from build123d import *

# Parameters (mm, degrees)
F1_DEPTH = 76.1175008
F2_R     = 1.98374
F3_R     = 3.69316
F4_R     = 1.8288
F5_DEPTH = 1.70942
F6_R     = 0.762
F7_W     = 6
F7_H     = 3.175
F8_DEPTH = 1.70942


# Not quite as in the source:
# - a feature names something its author has since deleted; it is built from what else it names


with BuildPart() as f1:
    # F0 (on Top) → F1 (new body)
    with BuildSketch(Plane.XY):
        Polygon((-1.70942, 0), (0, 0), (0, 16.7533828), (28.6143954, 16.7533828), (28.6143954, 31.2090308), (26.9049754, 31.2090308), (26.9049754, 18.4628028), (-1.70942, 18.4628028), align=None)
    extrude(amount=F1_DEPTH)

    # F2
    f2_edges = [f1.edges().sort_by_distance(p)[0] for p in [
        (0, 16.753383, 38.05875),
        (26.904975, 18.462803, 38.05875),
    ]]
    fillet(f2_edges, radius=F2_R)

    # F3
    f3_edges = [f1.edges().sort_by_distance(p)[0] for p in [
        (-1.70942, 18.462803, 38.05875),
        (28.614395, 16.753383, 38.05875),
    ]]
    fillet(f3_edges, radius=F3_R)

    # F4 (on face) → F5 (cut, through all)
    with BuildSketch(Plane.XZ.offset(-16.7533828)):
        with Locations((20.9524854, 72.1487508)):
            Circle(F4_R)
        with Locations((20.9524854, 38.0587504)):
            Circle(F4_R)
        with Locations((20.9524854, 3.96875)):
            Circle(F4_R)
    extrude(amount=-F5_DEPTH, mode=Mode.SUBTRACT)

    # F6
    f6_edges = [f1.edges().sort_by_distance(p)[0] for p in [
        (-0.85471, 0, 76.117501),
        (-0.85471, 0, 0),
    ]]
    fillet(f6_edges, radius=F6_R)

    # F7 (on face) → F8 (cut, through all)
    with BuildSketch(Plane(origin=(26.9049754, 0, 0), x_dir=(0, -1, 0), z_dir=(-1, 0, 0))):
        with Locations((-25.0340308, 71.3550008)):
            Rectangle(F7_W, F7_H)
        with Locations((-25.0340308, 4.7625)):
            Rectangle(F7_W, F7_H)
    extrude(amount=-F8_DEPTH, mode=Mode.SUBTRACT)


solid = f1.part
For this review, take the finished solid that the model builds, in its own axes (mm). A direction names the side the tool comes from. Give positions to 0.01 mm unless a question says otherwise; leave off trailing zeros. Order: outer loops, then holes, each group sorted by start corner. A loop starts at its lowest first (then second) coordinate and runs counter-clockwise, first axis right, second up. Notation, with made-up numbers: (-6, -19) - (40, -19) arc R16 ccw to (40, 5) - close; hole circle Ø10 at (-30.5, 42). An arc over 180 degrees is marked (long way). Answer as a JSON object with one key per item and string values. Group by question number.
Item 1: Take a section at D-D on x = 10.5. Give the boundary of the cut face in (y, z).
Item 2: Clearance check with flat-ended pins moving along their axes: pin 1 Ø1.9 at (x, z) = (28, 72) entering from -Y; pin 2 Ø5 at (x, y) = (15.5, 21.5) entering from +Z; pin 3 Ø11.5 at (x, z) = (16.5, 46) entering from +Y; pin 4 Ø5.5 at (y, z) = (26, 21.5) entering from -X (3 decimals). State where each tip first meets the part, or that it passes through.
Item 3: Take a section at A-A on x = 22. Give the boundary of the cut face in (y, z), and give its area (3 significant figures).
Item 4: Draft analysis for pull direction Y (two halves, no side actions). For faces 4 (the flat face through (28.614, 26, 38)), 5 (the flat face through (-1, 0, 38)), 6 (the flat face through (28, 25, 3.175)), state which applies: pulls with the +Y half, pulls with the -Y half, needs draft (parallel to the pull), parting line crosses it, or undercut.
Item 5: Wall thickness on line 1 along Z through (x, y) = (20, 17.5); line 2 along Y through (x, z) = (23.5, 51.5); line 3 along X through (y, z) = (14, 65): over which ranges is each line inside the solid? List them lowest first.
Item 6: Take a section at C-C on y = 7.5. Give the boundary of the cut face in (x, z).
Item 7: Machinability: for faces 1 (the flat face through (0, 7, 38)), 2 (the flat face through (14, 18.463, 38)), 3 (the flat face through (28, 25, 69.768)), which of the approach directions +Z, -Z, +X, -X, +Y, -Y give a long, thin tool a straight path to every point of the face, cutting with its end or side? Answer none if there is none.
Item 8: Take a section at B-B on z = 13.5. Give the boundary of the cut face in (x, y).
Reported:
{
 "1": {"outline": "(16.75, 0) - (18.46, 0) - (18.46, 76.12) - (16.75, 76.12) - close"},
 "2": {"pin 1": "y = 17.43", "pin 2": "through", "pin 3": "y = 18.46", "pin 4": "x = 26.905"},
 "3": {"outline": "(16.75, 0) - (18.46, 0) - (18.46, 2.47) - (16.75, 2.47) - close; (16.75, 5.47) - (18.46, 5.47) - (18.46, 36.56) - (16.75, 36.56) - close; (16.75, 39.56) - (18.46, 39.56) - (18.46, 70.65) - (16.75, 70.65) - close; (16.75, 73.65) - (18.46, 73.65) - (18.46, 76.12) - (16.75, 76.12) - close", "area": "115 mm^2"},
 "4": {"face 4": "needs draft", "face 5": "pulls with the -Y half", "face 6": "undercut"},
 "5": {"line 1": "0 to 2.41, 5.53 to 36.5, 39.62 to 70.59, 73.71 to 76.12", "line 2": "16.75 to 18.46", "line 3": "-1.71 to 0"},
 "6": {"outline": "(-1.71, 0) - (0, 0) - (0, 76.12) - (-1.71, 76.12) - close"},
 "7": {"face 1": "+Z, -Z, +X, -Y", "face 2": "+Z, -Z, -X, +Y", "face 3": "+X, -X"},
 "8": {"outline": "(-1.71, 0) - (0, 0) - (0, 14.77) arc R1.98 cw to (1.98, 16.75) - (24.92, 16.75) arc R3.69 ccw to (28.61, 20.45) - (28.61, 31.21) - (26.9, 31.21) - (26.9, 20.45) arc R1.98 cw to (24.92, 18.46) - (1.98, 18.46) arc R3.69 ccw to (-1.71, 14.77) - close"}
}
